Print and shaded views of the part. All mm, measured from the part's lowest x, y and z. Round coordinates to 2 decimals unless told otherwise and drop trailing zeros. Write each loop counter-clockwise with the first axis right and the second up, starting at its lowest first coordinate (ties: lowest second). Pieces come first, ordered by that corner, then holes. Notation, with made-up numbers: M 34.5,31 L 42.5,31 A18 ccw 42.5,57 Z; hole C 32,3.5 d7. An arc over 180 degrees is marked long. Write item = value, one per line. Start each with the question number.
Q1. Band-saw the part on C-C on y = 1.05. Write the cut outline in (x, z), plus the area to 3 significant figures.
Q2. Drop flat-ended pins along their axis: P1, Ø1, axis at x = 18, z = 13, coming from the -Y side; P2, Ø2.5, axis at x = 4.5, z = 17, coming from the +Y side. Give the stop position or say it passes through.
Q3. Probe L1, parallel to Z at x = 4.5, y = 1.95; L2, parallel to Z at x = 5.5, y = 2.3. List the from-to ranges inside material, lowest first.
Q4. Pull direction X, two halves, no side cores. Call the marked faces 1, 2 and 3: released by +X, released by -X, zero draft, split by the parting line, or undercut.
Q5. Band-saw the part on B-B on z = 4. Write the cut outline in (x, y), plus the area to 3 significant figures.
Q6. Band-saw the part on A-A on x = 4.5. Write the cut outline in (y, z), plus the area to 3 significant figures.
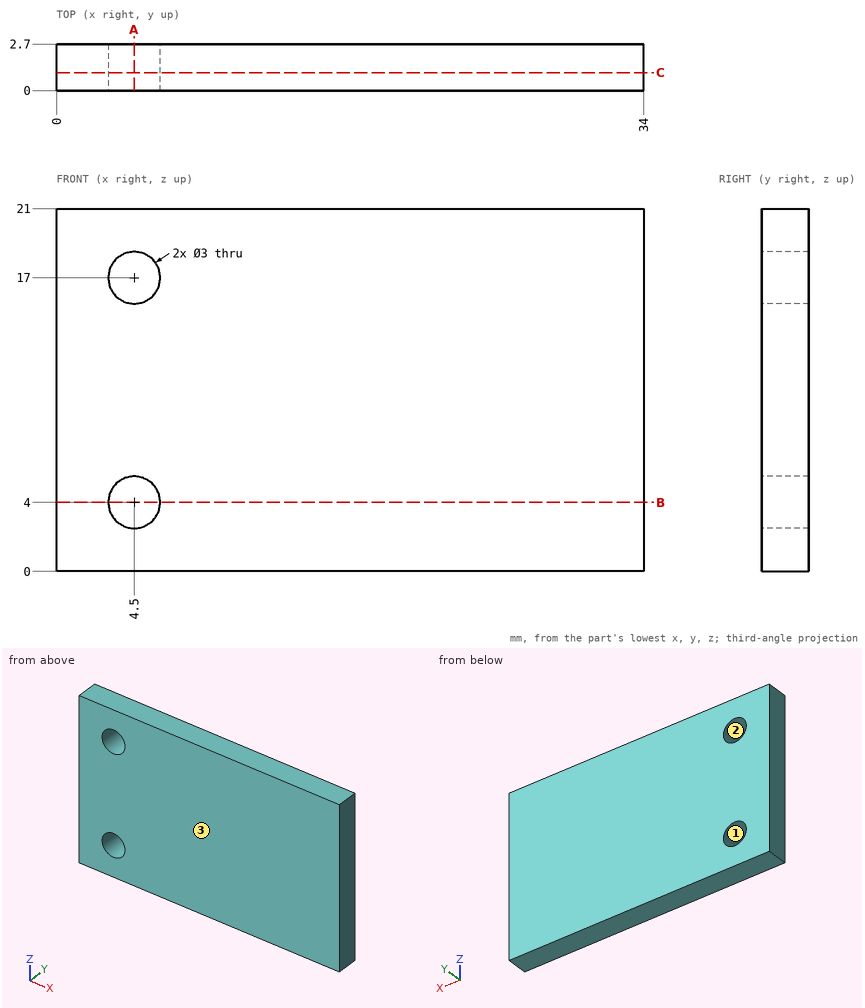
Conclusion:
q1.outline = M 0,0 L 34,0 L 34,21 L 0,21 Z; hole C 4.5,4 d3; hole C 4.5,17 d3
q1.area = 700 mm^2
q2.P1 = 0
q2.P2 = through
q3.L1 = 0 to 2.5, 5.5 to 15.5, 18.5 to 21
q3.L2 = 0 to 2.88, 5.12 to 15.88, 18.12 to 21
q4.face_1 = undercut
q4.face_2 = undercut
q4.face_3 = zero draft
q5.outline = M 0,0 L 3,0 L 3,2.7 L 0,2.7 Z; M 6,0 L 34,0 L 34,2.7 L 6,2.7 Z
q5.area = 83.7 mm^2
q6.outline = M 0,0 L 2.7,0 L 2.7,2.5 L 0,2.5 Z; M 0,5.5 L 2.7,5.5 L 2.7,15.5 L 0,15.5 Z; M 0,18.5 L 2.7,18.5 L 2.7,21 L 0,21 Z
q6.area = 40.5 mm^2
